The model under review builds one solid part; all positions refer to its coordinate system, in mm. A direction names the side the tool comes from. Coordinates: 2 decimals unless noted, no trailing zeros. Loops run counter-clockwise (first coordinate to the right, second up) from the corner with the lowest first, then second, coordinate; pieces in that order, holes last. Notation, with made-up numbers: (-3.75, 65) - (20.25, 65) arc R17 cw to (20.25, 93) - close; hole circle Ø3 at (11, 72). An arc over 180 degrees is marked (long way). Answer in a Markdown table with one row per item. Add a question column.
(1) We need section B-B on y = 125. Write out the cut boundary in (x, z), plus the area to 4 significant figures.
(2) For P1, Ø1.5, axis at x = 3, y = 152, coming from the +Z side; P2, Ø8, axis at y = 35, z = -100, coming from the +X side; P3, Ø6, axis at y = 53.25, z = -50, coming from the -X side; P4, Ø1.5, axis at x = 2.5, z = -164.5, coming from the -Y side, all flat-tipped, find the tip position at first contact; note any pin that passes through.
(3) We need section A-A on y = 35. Write out the cut boundary in (x, z), plus the area to 3 significant figures.
(4) For line 1 along Y through (x, z) = (1.4, -175); line 2 along Y through (x, z) = (2.25, -98); line 3 along Z through (x, y) = (0.6, 51.5), list the stretches that pass through material, from the lowest coordinate up.
(5) Machinability: for faces 1 (the flat face through (2, 0, -25)), 2 (the flat face through (2, 153, -157.5)), 3 (the flat face through (2, -3, -150)), which of the approach directions +Z, -Z, +X, -X, +Y, -Y give a long, thin tool a straight path to every point of the face, cutting with its end or side? Answer none if there is none.
(6) We need section C-C on x = 3.8. Give the number of separate pieces and of enclosed holes in the cut face, plus the area to 3 significant figures.
(7) We need section D-D on y = 53.25. Write out the cut boundary in (x, z) (3 decimals), plus the area to 3 significant figures.
from build123d import *

# Parameters (mm, degrees)
CROQUIS1_R              = 5
CROQUIS1_R_2            = 4
CROQUIS1_R_3            = 2.5
SALIENTE_EXTRUIR1_DEPTH = 5


with BuildPart() as part:
    # Croquis1 → Saliente-Extruir1 (new body)
    with BuildSketch(Plane(origin=(0, 0, 0), x_dir=(0, 0, -1), z_dir=(1, 0, 0))):
        Polygon((150, 150), (0, 50), (0, 0), (50, 0), (50, -5), (150, -5), (150, 0), (200, 0), (200, 150), (192.5, 150), (192.5, 155), (157.5, 155), (157.5, 150), align=None)
        with Locations((175, 125)):
            Circle(CROQUIS1_R, mode=Mode.SUBTRACT)
        with Locations((175, 20)):
            Circle(CROQUIS1_R_2, mode=Mode.SUBTRACT)
        with Locations((150, 35)):
            Circle(CROQUIS1_R_2, mode=Mode.SUBTRACT)
        with Locations((175, 143.25)):
            Circle(CROQUIS1_R_3, mode=Mode.SUBTRACT)
        with Locations((175, 106.75)):
            Circle(CROQUIS1_R_3, mode=Mode.SUBTRACT)
        with Locations((100, 35)):
            Circle(CROQUIS1_R, mode=Mode.SUBTRACT)
        with Locations((84.5, 60.685599078)):
            Circle(CROQUIS1_R_2, mode=Mode.SUBTRACT)
        with Locations((100, 53.25)):
            Circle(CROQUIS1_R_3, mode=Mode.SUBTRACT)
        with Locations((100, 16.75)):
            Circle(CROQUIS1_R_3, mode=Mode.SUBTRACT)
        with Locations((50, 35)):
            Circle(CROQUIS1_R, mode=Mode.SUBTRACT)
        with Locations((50, 53.25)):
            Circle(CROQUIS1_R_3, mode=Mode.SUBTRACT)
        with Locations((50, 16.75)):
            Circle(CROQUIS1_R_3, mode=Mode.SUBTRACT)
    extrude(amount=SALIENTE_EXTRUIR1_DEPTH)


solid = part.part
Outcome:
| question | item | result |
|---|---|---|
| 1 | outline | (0, -200) - (5, -200) - (5, -180) - (0, -180) - close; (0, -170) - (5, -170) - (5, -112.5) - (0, -112.5) - close |
| 1 | area | 387.5 mm² |
| 2 | P1 | z = -157.5 |
| 2 | P2 | through |
| 2 | P3 | x = 0 |
| 2 | P4 | y = 0 |
| 3 | outline | (0, -200) - (5, -200) - (5, -154) - (0, -154) - close; (0, -146) - (5, -146) - (5, -105) - (0, -105) - close; (0, -95) - (5, -95) - (5, -55) - (0, -55) - close; (0, -45) - (5, -45) - (5, 0) - (0, 0) - close |
| 3 | area | 860 mm² |
| 4 | line 1 | 0 to 16, 24 to 104.25, 109.25 to 120, 130 to 140.75, 145.75 to 155 |
| 4 | line 2 | -5 to 15.25, 18.25 to 30.42, 39.58 to 51.75, 54.75 to 115.33 |
| 4 | line 3 | -200 to -101.79, -98.21 to -51.79, -48.21 to -2.25 |
| 5 | face 1 | +Z, +X, -X, -Y |
| 5 | face 2 | +Z, +X, -X, +Y |
| 5 | face 3 | -Z, +X, -X, -Y |
| 6 | separate pieces | 1 |
| 6 | enclosed holes | 12 |
| 6 | area | 22,700 mm² |
| 7 | outline | (0, -200) - (5, -200) - (5, -102.5) - (0, -102.5) - close; (0, -97.5) - (5, -97.5) - (5, -52.5) - (0, -52.5) - close; (0, -47.5) - (5, -47.5) - (5, -4.875) - (0, -4.875) - close |
| 7 | area | 926 mm² |
